from build123d import *

# Parameters (mm, degrees)
CYLINDER423_R               = 3
CYLINDER423_DEPTH           = 4
CYLINDER422_R               = 3
CYLINDER422_DEPTH           = 4
CYLINDER420_R               = 3
CYLINDER420_DEPTH           = 4
CYLINDER421_R               = 3
CYLINDER421_DEPTH           = 4
COMPOUND319_PLACEMENT_ANGLE = 90
CYLINDER419_R               = 1.5
CYLINDER419_DEPTH           = 20
CYLINDER418_R               = 1.5
CYLINDER418_DEPTH           = 20
CYLINDER416_R               = 1.5
CYLINDER416_DEPTH           = 20
CYLINDER417_R               = 1.5
CYLINDER417_DEPTH           = 20
COMPOUND318_PLACEMENT_ANGLE = 90
CYLINDER309_R               = 1.5
CYLINDER309_DEPTH           = 50
CYLINDER310_R               = 1.5
CYLINDER310_DEPTH           = 50
CYLINDER307_R               = 3
CYLINDER307_DEPTH           = 4
CYLINDER308_R               = 3
CYLINDER308_DEPTH           = 4
PAD_DEPTH                   = 10


with BuildPart() as obj1:
    # Cylinder423 → Cylinder423 (new body)
    with BuildSketch(Plane(origin=(-7, -34, 37), x_dir=(1, 0, 0), z_dir=(0, -1, 0))):
        Circle(CYLINDER423_R)
    extrude(amount=CYLINDER423_DEPTH)


with BuildPart() as obj2:
    # Cylinder422 → Cylinder422 (new body)
    with BuildSketch(Plane(origin=(7, -34, 73), x_dir=(1, 0, 0), z_dir=(0, -1, 0))):
        Circle(CYLINDER422_R)
    extrude(amount=CYLINDER422_DEPTH)


with BuildPart() as obj3:
    # Cylinder420 → Cylinder420 (new body)
    with BuildSketch(Plane(origin=(-7, -34, 73), x_dir=(1, 0, 0), z_dir=(0, -1, 0))):
        Circle(CYLINDER420_R)
    extrude(amount=CYLINDER420_DEPTH)


with BuildPart() as compound319:
    # Cylinder421 → Cylinder421 (new body)
    with BuildSketch(Plane(origin=(7, -34, 37), x_dir=(1, 0, 0), z_dir=(0, -1, 0))):
        Circle(CYLINDER421_R)
    extrude(amount=CYLINDER421_DEPTH)

    # Compound319: union obj1, obj2, obj3
    add(obj1.part)
    add(obj2.part)
    add(obj3.part)


with BuildPart() as compound319_1:
    # Compound319 placement: moved
    add(compound319.part.moved(Location((0, 141, 45))).rotate(Axis((0, 141, 45), (1, 0, 0)), COMPOUND319_PLACEMENT_ANGLE))


with BuildPart() as obj4:
    # Cylinder419 → Cylinder419 (new body)
    with BuildSketch(Plane(origin=(-7, -34, 37), x_dir=(1, 0, 0), z_dir=(0, -1, 0))):
        Circle(CYLINDER419_R)
    extrude(amount=CYLINDER419_DEPTH)


with BuildPart() as obj5:
    # Cylinder418 → Cylinder418 (new body)
    with BuildSketch(Plane(origin=(7, -34, 73), x_dir=(1, 0, 0), z_dir=(0, -1, 0))):
        Circle(CYLINDER418_R)
    extrude(amount=CYLINDER418_DEPTH)


with BuildPart() as obj6:
    # Cylinder416 → Cylinder416 (new body)
    with BuildSketch(Plane(origin=(-7, -34, 73), x_dir=(1, 0, 0), z_dir=(0, -1, 0))):
        Circle(CYLINDER416_R)
    extrude(amount=CYLINDER416_DEPTH)


with BuildPart() as compound318:
    # Cylinder417 → Cylinder417 (new body)
    with BuildSketch(Plane(origin=(7, -34, 37), x_dir=(1, 0, 0), z_dir=(0, -1, 0))):
        Circle(CYLINDER417_R)
    extrude(amount=CYLINDER417_DEPTH)

    # Compound318: union obj4, obj5, obj6
    add(obj4.part)
    add(obj5.part)
    add(obj6.part)


with BuildPart() as compound318_1:
    # Compound318 placement: moved
    add(compound318.part.moved(Location((0, 141, 45))).rotate(Axis((0, 141, 45), (1, 0, 0)), COMPOUND318_PLACEMENT_ANGLE))


with BuildPart() as obj7:
    # Cylinder309 → Cylinder309 (new body)
    with BuildSketch(Plane(origin=(34, 36, 0), x_dir=(1, 0, 0), z_dir=(0, 0, 1))):
        Circle(CYLINDER309_R)
    extrude(amount=CYLINDER309_DEPTH)


with BuildPart() as compound289:
    # Cylinder310 → Cylinder310 (new body)
    with BuildSketch(Plane(origin=(-34, 36, 0), x_dir=(1, 0, 0), z_dir=(0, 0, 1))):
        Circle(CYLINDER310_R)
    extrude(amount=CYLINDER310_DEPTH)

    # Compound289: union obj7
    add(obj7.part)


with BuildPart() as obj8:
    # Cylinder307 → Cylinder307 (new body)
    with BuildSketch(Plane(origin=(-34, 36, -1), x_dir=(1, 0, 0), z_dir=(0, 0, 1))):
        Circle(CYLINDER307_R)
    extrude(amount=CYLINDER307_DEPTH)


with BuildPart() as compound288:
    # Cylinder308 → Cylinder308 (new body)
    with BuildSketch(Plane(origin=(34, 36, -1), x_dir=(1, 0, 0), z_dir=(0, 0, 1))):
        Circle(CYLINDER308_R)
    extrude(amount=CYLINDER308_DEPTH)

    # Compound288: union obj8
    add(obj8.part)


with BuildPart() as cut167:
    # Sketch → Pad (new body)
    with BuildSketch(Plane.XY):
        Polygon((-51.883896, 28.015725), (-8.825714, 110.528281), (8.883465, 110.528281), (51.774643, 28.198511), (0, 55.140807), align=None)
    extrude(amount=PAD_DEPTH)

    # Cut134: cut Compound288
    add(compound288.part, mode=Mode.SUBTRACT)

    # Cut135: cut Compound289
    add(compound289.part, mode=Mode.SUBTRACT)

    # Cut165: cut Compound318
    add(compound318_1.part, mode=Mode.SUBTRACT)

    # Cut167: cut Compound319
    add(compound319_1.part, mode=Mode.SUBTRACT)


solid = cut167.part
Work out the finished part from the listing and answer in its coordinate system (mm). A direction names the side the tool comes from. Round coordinates to 2 decimals unless told otherwise and drop trailing zeros. Write each loop counter-clockwise with the first axis right and the second up, starting at its lowest first coordinate (ties: lowest second). Pieces come first, ordered by that corner, then holes. Notation, with made-up numbers: M 35,78.5 L 73,78.5 A26 ccw 73,111.5 Z; hole C 88,84 d7. An arc over 180 degrees is marked long. Use a Markdown table: item, result.
1) The part is cut by section A-A on x = -7. Give the vertices of the cut face in (y, z).
Taken from the geometry:
| item | result |
|---|---|
| outline | M 51.48,0 L 66.5,0 L 66.5,7 L 65,7 L 65,10 L 51.48,10 Z; M 69.5,0 L 102.5,0 L 102.5,7 L 101,7 L 101,10 L 71,10 L 71,7 L 69.5,7 Z; M 105.5,0 L 110.53,0 L 110.53,10 L 107,10 L 107,7 L 105.5,7 Z |
2) Flat-ended cylindrical pins translate along their axes: pin 1 (5 mm diameter, centred on x = -7, y = 104, fed in from -Z); pin 2 (4 mm diameter, centred on x = -7, y = 68, fed in from +Z); pin 3 (5 mm diameter, centred on y = 50.5, z = 8, fed in from -X); pin 4 (5 mm diameter, centred on x = -29.5, z = 1.5, fed in from -Y). Find the tip coordinate at first contact, or state that the pin passes through.
Taken from the geometry:
| item | result |
|---|---|
| pin 1 | stops at z = 0 |
| pin 2 | stops at z = 7 |
| pin 3 | stops at x = -41.46 |
| pin 4 | stops at y = 38.41 |
3) Determine the mould class of faces 1 (the face through (-30.66, 68.69, 4.93)), 2 (the face through (-5.616, 70.662, 8.521)), 3 (the face through (1, 70, 0)) for opening direction X: pulls with the +X half, pulls with the -X half, needs draft (parallel to the pull), parting line crosses it, or undercut.
Taken from the geometry:
| item | result |
|---|---|
| face 1 | pulls with the -X half |
| face 2 | undercut |
| face 3 | needs draft |
4) The part is cut by section B-B on y = 54. Give the vertices of the cut face in (x, z), plus the area to 3 significant figures.
Taken from the geometry:
| item | result |
|---|---|
| outline | M -38.32,0 L -2.18,0 L -2.18,10 L -38.32,10 Z; M 2.19,0 L 38.33,0 L 38.33,10 L 2.19,10 Z |
| area | 723 mm2 |
5) The part is cut by section C-C on z = 4.5. Give the vertices of the cut face in (x, y), plus the area to 3 significant figures.
Taken from the geometry:
| item | result |
|---|---|
| outline | M -51.88,28.02 L -35.35,36.66 A1.5 cw -33.78,37.48 L 0,55.14 L 33.91,37.5 A1.5 cw 35.28,36.78 L 51.77,28.2 L 8.88,110.53 L -8.83,110.53 Z; hole C -7,68 d3; hole C -7,104 d3; hole C 7,68 d3; hole C 7,104 d3 |
| area | 3,570 mm2 |
6) The part is cut by section D-D on y = 104. Give the vertices of the cut face in (x, z).
Taken from the geometry:
| item | result |
|---|---|
| outline | M -12.23,0 L -8.5,0 L -8.5,7 L -10,7 L -10,10 L -12.23,10 Z; M -5.5,0 L 5.5,0 L 5.5,7 L 4,7 L 4,10 L -4,10 L -4,7 L -5.5,7 Z; M 8.5,0 L 12.28,0 L 12.28,10 L 10,10 L 10,7 L 8.5,7 Z |
7) Consider line 1 (X direction, y = 68, z = 8.7); line 2 (Y direction, x = 7, z = 9.2); line 3 (Y direction, x = 7, z = 4.75). Determine where each line is inside the solid, lowest interval first. Write a range as [from, to].
Taken from the geometry:
| item | result |
|---|---|
| line 1 | x = [-31.02, -10], [-4, 4], [10, 31.04] |
| line 2 | y = [51.5, 65], [71, 101], [107, 110.53] |
| line 3 | y = [51.5, 66.5], [69.5, 102.5], [105.5, 110.53] |
8) Which of the six approach directions +Z, -Z, +X, -X, +Y, -Y give full straight-line access (tool end or side, diameter ignored) to faces 4 (the face through (35, 38, 3)), 5 (the face through (17.19, 46.195, 4.93)), 6 (the face through (-6.194, 66.735, 3.549)), 7 (the face through (-5.7, 105.3, 7))?
Taken from the geometry:
| item | result |
|---|---|
| face 4 | -Z, -Y |
| face 5 | +Z, -Z, -Y |
| face 6 | +Z, -Z |
| face 7 | +Z |
